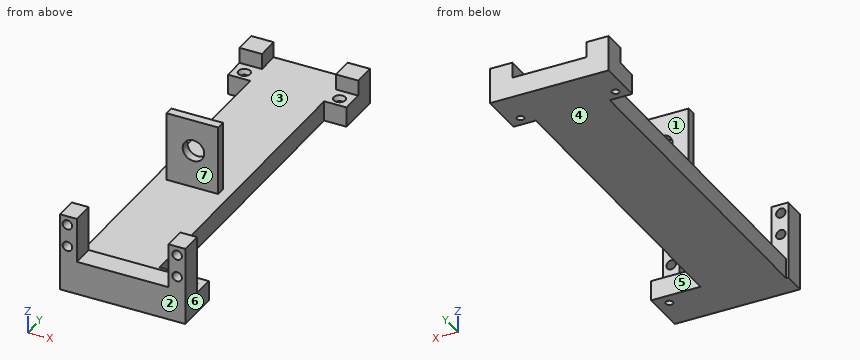
from build123d import *

# Parameters (mm, degrees)
CYLINDER148_R     = 4.8
CYLINDER148_DEPTH = 6.7
CYLINDER147_R     = 1.6
CYLINDER147_DEPTH = 7
CYLINDER146_R     = 1.6
CYLINDER146_DEPTH = 7
CYLINDER140_R     = 1.6
CYLINDER140_DEPTH = 7
CYLINDER012_R     = 2.125
CYLINDER012_DEPTH = 10
CYLINDER013_R     = 2.125
CYLINDER013_DEPTH = 10
CYLINDER010_R     = 2.125
CYLINDER010_DEPTH = 10
CYLINDER011_R     = 2.125
CYLINDER011_DEPTH = 10
CYLINDER145_R     = 3.45
CYLINDER145_DEPTH = 10
CYLINDER141_R     = 1.6
CYLINDER141_DEPTH = 7
CYLINDER142_R     = 1.6
CYLINDER142_DEPTH = 7
CYLINDER144_R     = 1.6
CYLINDER144_DEPTH = 7
CYLINDER143_R     = 1.6
CYLINDER143_DEPTH = 7
BOX007_W          = 41
BOX007_H          = 10
BOX007_DEPTH      = 20
BOX006_W          = 56
BOX006_H          = 10
BOX006_DEPTH      = 26
BOX005_W          = 23
BOX005_H          = 4
BOX005_DEPTH      = 31
BOX008_W          = 22
BOX008_H          = 10
BOX008_DEPTH      = 9
BOX009_W          = 1
BOX009_H          = 10
BOX009_DEPTH      = 9
BOX012_W          = 10
BOX012_H          = 10
BOX012_DEPTH      = 16
BOX013_W          = 10
BOX013_H          = 10
BOX013_DEPTH      = 16
BOX014_W          = 22
BOX014_H          = 10
BOX014_DEPTH      = 9
BOX015_W          = 10
BOX015_H          = 10
BOX015_DEPTH      = 9
BOX016_W          = 10
BOX016_H          = 10
BOX016_DEPTH      = 9
BOX003_W          = 33
BOX003_H          = 180.5
BOX003_DEPTH      = 9


with BuildPart() as hole002:
    # Cylinder148 → Cylinder148 (new body)
    with BuildSketch(Plane(origin=(18, 73, 20), x_dir=(1, 0, 0), z_dir=(0, -1, 0))):
        Circle(CYLINDER148_R)
    extrude(amount=CYLINDER148_DEPTH)


with BuildPart() as wheelscrew018:
    # Cylinder147 → Cylinder147 (new body)
    with BuildSketch(Plane(origin=(9, -124, -19), x_dir=(1, 0, 0), z_dir=(0, 0, 1))):
        Circle(CYLINDER147_R)
    extrude(amount=CYLINDER147_DEPTH)


with BuildPart() as obj1:
    # Cone015 → Cone015 (revolve)
    with BuildSketch(Plane(origin=(9, -124, -12), x_dir=(1, 0, 0), z_dir=(0, -1, 0))):
        Polygon((0, 0), (1.6, 0), (2.65, 2), (0, 2), align=None)
    revolve(axis=Axis((9, -124, -12), (0, 0, 1)))

    # Fusion007051: union wheelScrew018
    add(wheelscrew018.part)


with BuildPart() as obj1_1:
    # Fusion007051 placement: moved
    add(obj1.part.moved(Location((41.5, 128.5, 13))))


with BuildPart() as wheelscrew016:
    # Cylinder146 → Cylinder146 (new body)
    with BuildSketch(Plane(origin=(9, -124, -19), x_dir=(1, 0, 0), z_dir=(0, 0, 1))):
        Circle(CYLINDER146_R)
    extrude(amount=CYLINDER146_DEPTH)


with BuildPart() as obj2:
    # Cone014 → Cone014 (revolve)
    with BuildSketch(Plane(origin=(9, -124, -12), x_dir=(1, 0, 0), z_dir=(0, -1, 0))):
        Polygon((0, 0), (1.6, 0), (2.65, 2), (0, 2), align=None)
    revolve(axis=Axis((9, -124, -12), (0, 0, 1)))

    # Fusion007050: union wheelScrew016
    add(wheelscrew016.part)


with BuildPart() as obj2_1:
    # Fusion007050 placement: moved
    add(obj2.part.moved(Location((-13, 278.5, 13))))


with BuildPart() as wheelscrew005:
    # Cylinder140 → Cylinder140 (new body)
    with BuildSketch(Plane(origin=(9, -124, -19), x_dir=(1, 0, 0), z_dir=(0, 0, 1))):
        Circle(CYLINDER140_R)
    extrude(amount=CYLINDER140_DEPTH)


with BuildPart() as obj3:
    # Cone009 → Cone009 (revolve)
    with BuildSketch(Plane(origin=(9, -124, -12), x_dir=(1, 0, 0), z_dir=(0, -1, 0))):
        Polygon((0, 0), (1.6, 0), (2.65, 2), (0, 2), align=None)
    revolve(axis=Axis((9, -124, -12), (0, 0, 1)))

    # Fusion007043: union wheelScrew005
    add(wheelscrew005.part)


with BuildPart() as obj3_1:
    # Fusion007043 placement: moved
    add(obj3.part.moved(Location((29.5, 278.5, 13))))


with BuildPart() as servoattach003:
    # Cylinder012 → Cylinder012 (new body)
    with BuildSketch(Plane(origin=(52.3, -10.5, 25), x_dir=(1, 0, 0), z_dir=(0, 1, 0))):
        Circle(CYLINDER012_R)
    extrude(amount=CYLINDER012_DEPTH)


with BuildPart() as servoattach004:
    # Cylinder013 → Cylinder013 (new body)
    with BuildSketch(Plane(origin=(52.3, -10.5, 15), x_dir=(1, 0, 0), z_dir=(0, 1, 0))):
        Circle(CYLINDER013_R)
    extrude(amount=CYLINDER013_DEPTH)


with BuildPart() as servoattach001:
    # Cylinder010 → Cylinder010 (new body)
    with BuildSketch(Plane(origin=(3.3, -10.5, 25), x_dir=(1, 0, 0), z_dir=(0, 1, 0))):
        Circle(CYLINDER010_R)
    extrude(amount=CYLINDER010_DEPTH)


with BuildPart() as servoattach002:
    # Cylinder011 → Cylinder011 (new body)
    with BuildSketch(Plane(origin=(3.3, -10.5, 15), x_dir=(1, 0, 0), z_dir=(0, 1, 0))):
        Circle(CYLINDER011_R)
    extrude(amount=CYLINDER011_DEPTH)


with BuildPart() as insert001:
    # Cylinder145 → Cylinder145 (new body)
    with BuildSketch(Plane(origin=(17.5, 180.5, -7), x_dir=(1, 0, 0), z_dir=(0, 0, 1))):
        Circle(CYLINDER145_R)
    extrude(amount=CYLINDER145_DEPTH)


with BuildPart() as wheelscrew008:
    # Cylinder141 → Cylinder141 (new body)
    with BuildSketch(Plane(origin=(9, -124, -19), x_dir=(1, 0, 0), z_dir=(0, 0, 1))):
        Circle(CYLINDER141_R)
    extrude(amount=CYLINDER141_DEPTH)


with BuildPart() as obj4:
    # Cone010 → Cone010 (revolve)
    with BuildSketch(Plane(origin=(9, -124, -12), x_dir=(1, 0, 0), z_dir=(0, -1, 0))):
        Polygon((0, 0), (1.6, 0), (2.65, 2), (0, 2), align=None)
    revolve(axis=Axis((9, -124, -12), (0, 0, 1)))

    # Fusion007045: union wheelScrew008
    add(wheelscrew008.part)


with BuildPart() as obj4_1:
    # Fusion007045 placement: moved
    add(obj4.part.moved(Location((17, 318, 13))))


with BuildPart() as wheelscrew010:
    # Cylinder142 → Cylinder142 (new body)
    with BuildSketch(Plane(origin=(9, -124, -19), x_dir=(1, 0, 0), z_dir=(0, 0, 1))):
        Circle(CYLINDER142_R)
    extrude(amount=CYLINDER142_DEPTH)


with BuildPart() as obj5:
    # Cone011 → Cone011 (revolve)
    with BuildSketch(Plane(origin=(9, -124, -12), x_dir=(1, 0, 0), z_dir=(0, -1, 0))):
        Polygon((0, 0), (1.6, 0), (2.65, 2), (0, 2), align=None)
    revolve(axis=Axis((9, -124, -12), (0, 0, 1)))

    # Fusion007046: union wheelScrew010
    add(wheelscrew010.part)


with BuildPart() as obj5_1:
    # Fusion007046 placement: moved
    add(obj5.part.moved(Location((-1, 318, 13))))


with BuildPart() as wheelscrew014:
    # Cylinder144 → Cylinder144 (new body)
    with BuildSketch(Plane(origin=(9, -124, -19), x_dir=(1, 0, 0), z_dir=(0, 0, 1))):
        Circle(CYLINDER144_R)
    extrude(amount=CYLINDER144_DEPTH)


with BuildPart() as obj6:
    # Cone013 → Cone013 (revolve)
    with BuildSketch(Plane(origin=(9, -124, -12), x_dir=(1, 0, 0), z_dir=(0, -1, 0))):
        Polygon((0, 0), (1.6, 0), (2.65, 2), (0, 2), align=None)
    revolve(axis=Axis((9, -124, -12), (0, 0, 1)))

    # Fusion007048: union wheelScrew014
    add(wheelscrew014.part)


with BuildPart() as obj6_1:
    # Fusion007048 placement: moved
    add(obj6.part.moved(Location((17, 88, 13))))


with BuildPart() as wheelscrew012:
    # Cylinder143 → Cylinder143 (new body)
    with BuildSketch(Plane(origin=(9, -124, -19), x_dir=(1, 0, 0), z_dir=(0, 0, 1))):
        Circle(CYLINDER143_R)
    extrude(amount=CYLINDER143_DEPTH)


with BuildPart() as obj7:
    # Cone012 → Cone012 (revolve)
    with BuildSketch(Plane(origin=(9, -124, -12), x_dir=(1, 0, 0), z_dir=(0, -1, 0))):
        Polygon((0, 0), (1.6, 0), (2.65, 2), (0, 2), align=None)
    revolve(axis=Axis((9, -124, -12), (0, 0, 1)))

    # Fusion007047: union wheelScrew012
    add(wheelscrew012.part)


with BuildPart() as obj7_1:
    # Fusion007047 placement: moved
    add(obj7.part.moved(Location((-1, 88, 13))))


with BuildPart() as frame005:
    # Box007 → Box007 (new body)
    with BuildSketch(Plane(origin=(7.5, -10.5, 9), x_dir=(1, 0, 0), z_dir=(0, 0, 1))):
        with Locations((20.5, 5)):
            Rectangle(BOX007_W, BOX007_H)
    extrude(amount=BOX007_DEPTH)


with BuildPart() as cut005:
    # Box006 → Box006 (new body)
    with BuildSketch(Plane(origin=(0, -10.5, 3), x_dir=(1, 0, 0), z_dir=(0, 0, 1))):
        with Locations((28, 5)):
            Rectangle(BOX006_W, BOX006_H)
    extrude(amount=BOX006_DEPTH)

    # Cut005: cut frame005
    add(frame005.part, mode=Mode.SUBTRACT)


with BuildPart() as frame003:
    # Box005 → Box005 (new body)
    with BuildSketch(Plane(origin=(6, 69, 3), x_dir=(1, 0, 0), z_dir=(0, 0, 1))):
        with Locations((11.5, 2)):
            Rectangle(BOX005_W, BOX005_H)
    extrude(amount=BOX005_DEPTH)


with BuildPart() as frame006:
    # Box008 → Box008 (new body)
    with BuildSketch(Plane(origin=(34, -10.5, -6), x_dir=(1, 0, 0), z_dir=(0, 0, 1))):
        with Locations((11, 5)):
            Rectangle(BOX008_W, BOX008_H)
    extrude(amount=BOX008_DEPTH)


with BuildPart() as frame007:
    # Box009 → Box009 (new body)
    with BuildSketch(Plane(origin=(0, -10.5, -6), x_dir=(1, 0, 0), z_dir=(0, 0, 1))):
        with Locations((0.5, 5)):
            Rectangle(BOX009_W, BOX009_H)
    extrude(amount=BOX009_DEPTH)


with BuildPart() as frame008:
    # Box012 → Box012 (new body)
    with BuildSketch(Plane(origin=(34, 160, -6), x_dir=(1, 0, 0), z_dir=(0, 0, 1))):
        with Locations((5, 5)):
            Rectangle(BOX012_W, BOX012_H)
    extrude(amount=BOX012_DEPTH)


with BuildPart() as frame009:
    # Box013 → Box013 (new body)
    with BuildSketch(Plane(origin=(-9, 160, -6), x_dir=(1, 0, 0), z_dir=(0, 0, 1))):
        with Locations((5, 5)):
            Rectangle(BOX013_W, BOX013_H)
    extrude(amount=BOX013_DEPTH)


with BuildPart() as frame010:
    # Box014 → Box014 (new body)
    with BuildSketch(Plane(origin=(34, -0.5, -6), x_dir=(1, 0, 0), z_dir=(0, 0, 1))):
        with Locations((11, 5)):
            Rectangle(BOX014_W, BOX014_H)
    extrude(amount=BOX014_DEPTH)


with BuildPart() as frame011:
    # Box015 → Box015 (new body)
    with BuildSketch(Plane(origin=(34, 150, -6), x_dir=(1, 0, 0), z_dir=(0, 0, 1))):
        with Locations((5, 5)):
            Rectangle(BOX015_W, BOX015_H)
    extrude(amount=BOX015_DEPTH)


with BuildPart() as frame012:
    # Box016 → Box016 (new body)
    with BuildSketch(Plane(origin=(-9, 150, -6), x_dir=(1, 0, 0), z_dir=(0, 0, 1))):
        with Locations((5, 5)):
            Rectangle(BOX016_W, BOX016_H)
    extrude(amount=BOX016_DEPTH)


with BuildPart() as base004:
    # Box003 → Box003 (new body)
    with BuildSketch(Plane(origin=(1, -10.5, -6), x_dir=(1, 0, 0), z_dir=(0, 0, 1))):
        with Locations((16.5, 90.25)):
            Rectangle(BOX003_W, BOX003_H)
    extrude(amount=BOX003_DEPTH)

    # Fusion007049: union Cut005, frame003, frame006, frame007, frame008, frame009, frame010, frame011, frame012
    add(cut005.part)
    add(frame003.part)
    add(frame006.part)
    add(frame007.part)
    add(frame008.part)
    add(frame009.part)
    add(frame010.part)
    add(frame011.part)
    add(frame012.part)

    # Cut006: cut obj7
    add(obj7_1.part, mode=Mode.SUBTRACT)

    # Cut007: cut obj6
    add(obj6_1.part, mode=Mode.SUBTRACT)

    # Cut008: cut obj5
    add(obj5_1.part, mode=Mode.SUBTRACT)

    # Cut009: cut obj4
    add(obj4_1.part, mode=Mode.SUBTRACT)

    # Cut010: cut insert001
    add(insert001.part, mode=Mode.SUBTRACT)

    # Cut011: cut servoAttach002
    add(servoattach002.part, mode=Mode.SUBTRACT)

    # Cut012: cut servoAttach001
    add(servoattach001.part, mode=Mode.SUBTRACT)

    # Cut013: cut servoAttach004
    add(servoattach004.part, mode=Mode.SUBTRACT)

    # Cut014: cut servoAttach003
    add(servoattach003.part, mode=Mode.SUBTRACT)

    # Cut015: cut obj3
    add(obj3_1.part, mode=Mode.SUBTRACT)

    # Cut016: cut obj2
    add(obj2_1.part, mode=Mode.SUBTRACT)

    # Cut017: cut obj1
    add(obj1_1.part, mode=Mode.SUBTRACT)

    # Cut018: cut hole002
    add(hole002.part, mode=Mode.SUBTRACT)


solid = base004.part
Model file for the job. Use its own axes, mm. Face numbers are marked on the shaded views. A direction names the side the tool comes from. Round coordinates to 2 decimals unless told otherwise and drop trailing zeros. Loops run counter-clockwise (first coordinate to the right, second up) from the corner with the lowest first, then second, coordinate; pieces in that order, holes last. Notation, with made-up numbers: (57, 81) -> (113, 81) arc R17 cw to (113, 90) -> close; hole circle Ø8 at (0, -8.75). An arc over 180 degrees is marked (long way). Answer as CSV lines item,"result". Start each with the question number.
1) Slice it at B-B (x = 38.5). List the corners of the cut face in (y, z).
2) Slice it at C-C (x = -4). List the corners of the cut face in (y, z), plus the area to 3 significant figures.
3) Mould opens along Y. For the marked faces 1, 2, 3 and 4 say: +Y half, -Y half, draft (parallel to the pull), parting line (faces both ways), or undercut.
4) Pin check, flat tips, straight feed: P1, Ø8, axis at y = 102.5, z = 3, coming from the -X side; P2, Ø2, axis at y = 71, z = 14.5, coming from the +X side; P3, Ø1.2, axis at y = 70.5, z = 16, coming from the -X side. Stop position of each tip, or through.
5) Tool access for the marked faces 5, 6 and 7: list every direction of +Z, -Z, +X, -X, +Y, -Y with a clear straight run to the whole face (end or side of a thin tool).
6) Slice it at A-A (y = 154.5). List the corners of the cut face in (x, z).
7) Slice it at D-D (z = 32). List the corners of the cut face in (x, y), plus the area to 3 significant figures.
8) Probe line 1 along Z through (x, y) = (52, -8); line 2 along X through (y, z) = (-6, 25) (3 decimals); line 3 along X through (y, z) = (154.5, -0.5). List the from-to ranges inside material, lowest first.
Filled in:
1,outline,"(-10.5, -6) -> (9.5, -6) -> (9.5, 3) -> (-0.5, 3) -> (-0.5, 9) -> (-10.5, 9) -> close; (150, -6) -> (152.9, -6) -> (152.9, 1) -> (151.85, 3) -> (150, 3) -> close; (156.1, -6) -> (170, -6) -> (170, 10) -> (160, 10) -> (160, 3) -> (157.15, 3) -> (156.1, 1) -> close"
2,outline,"(150, -6) -> (152.9, -6) -> (152.9, 1) -> (151.85, 3) -> (150, 3) -> close; (156.1, -6) -> (170, -6) -> (170, 10) -> (160, 10) -> (160, 3) -> (157.15, 3) -> (156.1, 1) -> close"
2,area,"219 mm2"
3,face 1,"+Y half"
3,face 2,"-Y half"
3,face 3,"undercut"
3,face 4,"draft"
4,P1,"stops at x = 1"
4,P2,"stops at x = 29"
4,P3,"stops at x = 6"
5,face 5,"+Z, -Z, +X"
5,face 6,"+Z, -Z, +X, +Y, -Y"
5,face 7,"+Z, +X, -X"
6,outline,"(-9, -6) -> (-5.6, -6) -> (-5.6, 1) -> (-6.65, 3) -> (-9, 3) -> close; (-2.4, -6) -> (36.9, -6) -> (36.9, 1) -> (35.85, 3) -> (-1.35, 3) -> (-2.4, 1) -> close; (40.1, -6) -> (44, -6) -> (44, 3) -> (41.15, 3) -> (40.1, 1) -> close"
7,outline,"(6, 69) -> (29, 69) -> (29, 73) -> (6, 73) -> close"
7,area,"92.0 mm2"
8,line 1,"z = -6 to 12.9, 17.1 to 22.9, 27.1 to 29"
8,line 2,"x = 0 to 1.175, 5.425 to 7.5, 48.5 to 50.175, 54.425 to 56"
8,line 3,"x = -9 to -5.6, -2.4 to 36.9, 40.1 to 44"
